from build123d import *

# Parameters (mm, degrees)
SKETCH_1_R          = 1.7
SKETCH_1_W          = 5
SKETCH_1_H          = 13
SKETCH_1_H_2        = 2
EXTRUDE_3_DEPTH     = 2.9
SKETCH_3_R          = 2.1
CUT_EXTRUDE_3_DEPTH = 2.9
SKETCH_4_W          = 20
SKETCH_4_H          = 40
SKETCH_4_R          = 2.1
EXTRUDE_4_DEPTH     = 2.9
SKETCH_5_W          = 70
SKETCH_5_H          = 40
SKETCH_5_W_2        = 69.6
SKETCH_5_H_2        = 39.6
CUT_EXTRUDE_4_DEPTH = 2.9


with BuildPart() as part:
    # 草图1 → 凸台-拉伸3 (new body)
    # profile 1 of 10: a face of its own
    with BuildSketch(Plane(origin=(0, 0, 0), x_dir=(1, 0, 0), z_dir=(0, 1, 0))):
        with BuildLine():
            Line((-40, 113), (-70, 113))
            Line((-70, 113), (-70, 108))
            Line((-70, 108), (-70, 92))
            Line((-70, 92), (-63.7, 92))
            ThreePointArc((-63.7, 92), (-62, 93.7), (-60.3, 92))
            ThreePointArc((-60.3, 92), (-60.797918472, 90.797918472), (-62, 90.3))
            Line((-62, 90.3), (-62, 87))
            Line((-62, 87), (-48, 87))
            Line((-48, 87), (-48, 90.3))
            ThreePointArc((-48, 90.3), (-49.202081528, 93.202081528), (-46.3, 92))
            Line((-46.3, 92), (-40, 92))
            Line((-40, 92), (-40, 113))
        make_face()
        with Locations(Location((-62, 108, 0), (0, 0, 270))):
            Circle(SKETCH_1_R, mode=Mode.SUBTRACT)
        with Locations(Location((-48, 108, 0), (0, 0, 270))):
            Circle(SKETCH_1_R, mode=Mode.SUBTRACT)
    # profile 2 of 10: a face of its own
    with BuildSketch(Plane(origin=(0, 0, 0), x_dir=(1, 0, 0), z_dir=(0, 1, 0))):
        with BuildLine():
            Line((-70, 92), (-70, 87))
            Line((-70, 87), (-62, 87))
            Line((-62, 87), (-62, 90.3))
            ThreePointArc((-62, 90.3), (-63.202081528, 90.797918472), (-63.7, 92))
            Line((-63.7, 92), (-70, 92))
        make_face()
    # profile 3 of 10: a face of its own
    with BuildSketch(Plane(origin=(0, 0, 0), x_dir=(1, 0, 0), z_dir=(0, 1, 0))):
        with BuildLine():
            Line((-48, 90.3), (-48, 87))
            Line((-48, 87), (-40, 87))
            Line((-40, 87), (-40, 92))
            Line((-40, 92), (-46.3, 92))
            ThreePointArc((-46.3, 92), (-46.797918472, 90.797918472), (-48, 90.3))
        make_face()
    # profile 4 of 10: a face of its own
    with BuildSketch(Plane(origin=(0, 0, 0), x_dir=(1, 0, 0), z_dir=(0, 1, 0))):
        Polygon((-70, 87), (-70, 80), (-20, 80), (-20, 85), (-25, 85), (-25, 87), (-40, 87), (-48, 87), (-62, 87), align=None)
    # profile 5 of 10: a face of its own
    with BuildSketch(Plane(origin=(0, 0, 0), x_dir=(1, 0, 0), z_dir=(0, 1, 0))):
        Polygon((-25, 113), (-40, 113), (-40, 92), (-40, 87), (-25, 87), (-25, 100), align=None)
    # profile 6 of 10: a face of its own
    with BuildSketch(Plane(origin=(0, 0, 0), x_dir=(1, 0, 0), z_dir=(0, 1, 0))):
        with Locations((-22.5, 93.5)):
            Rectangle(SKETCH_1_W, SKETCH_1_H)
    # profile 7 of 10: a face of its own
    with BuildSketch(Plane(origin=(0, 0, 0), x_dir=(1, 0, 0), z_dir=(0, 1, 0))):
        with Locations((-22.5, 106.5)):
            Rectangle(SKETCH_1_W, SKETCH_1_H)
    # profile 8 of 10: a face of its own
    with BuildSketch(Plane(origin=(0, 0, 0), x_dir=(1, 0, 0), z_dir=(0, 1, 0))):
        with Locations((-22.5, 86)):
            Rectangle(SKETCH_1_W, SKETCH_1_H_2)
    # profile 9 of 10: a face of its own
    with BuildSketch(Plane(origin=(0, 0, 0), x_dir=(1, 0, 0), z_dir=(0, 1, 0))):
        Polygon((-20, 120), (-70, 120), (-70, 113), (-40, 113), (-25, 113), (-25, 115), (-20, 115), align=None)
    # profile 10 of 10: a face of its own
    with BuildSketch(Plane(origin=(0, 0, 0), x_dir=(1, 0, 0), z_dir=(0, 1, 0))):
        with Locations((-22.5, 114)):
            Rectangle(SKETCH_1_W, SKETCH_1_H_2)
    extrude(amount=EXTRUDE_3_DEPTH)

    # 草图3 → 切除-拉伸3 (cut)
    with BuildSketch(Plane(origin=(0, 2.9, 0), x_dir=(1, 0, 0), z_dir=(0, 1, 0))):
        with Locations(Location((-25, 110, 0), (0, 0, 270))):
            Circle(SKETCH_3_R)
        with Locations(Location((-25, 90, 0), (0, 0, 270))):
            Circle(SKETCH_3_R)
        with Locations(Location((-35, 90, 0), (0, 0, 270))):
            Circle(SKETCH_3_R)
        with Locations(Location((-35, 110, 0), (0, 0, 270))):
            Circle(SKETCH_3_R)
    extrude(amount=-CUT_EXTRUDE_3_DEPTH, mode=Mode.SUBTRACT)

    # 草图4 → 凸台-拉伸4 (add)
    with BuildSketch(Plane(origin=(0, 2.9, 0), x_dir=(1, 0, 0), z_dir=(0, 1, 0))):
        with Locations((-10, 100)):
            Rectangle(SKETCH_4_W, SKETCH_4_H)
        with Locations(Location((-15, 110, 0), (0, 0, 270))):
            Circle(SKETCH_4_R, mode=Mode.SUBTRACT)
        with Locations(Location((-15, 90, 0), (0, 0, 270))):
            Circle(SKETCH_4_R, mode=Mode.SUBTRACT)
        with Locations(Location((-5, 110, 0), (0, 0, 270))):
            Circle(SKETCH_4_R, mode=Mode.SUBTRACT)
        with Locations(Location((-5, 90, 0), (0, 0, 270))):
            Circle(SKETCH_4_R, mode=Mode.SUBTRACT)
    extrude(amount=-EXTRUDE_4_DEPTH)

    # 草图5 → 切除-拉伸4 (cut)
    with BuildSketch(Plane(origin=(0, 2.9, 0), x_dir=(1, 0, 0), z_dir=(0, 1, 0))):
        with Locations((-35, 100)):
            Rectangle(SKETCH_5_W, SKETCH_5_H)
        with Locations((-35, 100)):
            Rectangle(SKETCH_5_W_2, SKETCH_5_H_2, mode=Mode.SUBTRACT)
    extrude(amount=-CUT_EXTRUDE_4_DEPTH, mode=Mode.SUBTRACT)


solid = part.part
CAD build for the part. Positions are in the model's coordinates, mm. Coordinates: 2 decimals unless noted, no trailing zeros. Order: outer loops, then holes, each group sorted by start corner. A loop starts at its lowest first (then second) coordinate and runs counter-clockwise, first axis right, second up.
Item 1: Two-plate mould, pull along X, no slides. Class faces 1 (the face through (-36.278, 1.47, -91.666)), 2 (the face through (-35, 2.9, -100)), 3 (the face through (-0.2, 1, -100)): +X half, -X half, draft (parallel to the pull), parting line (faces both ways), or undercut.
Check sheet entries:
face 1: undercut
face 2: draft
face 3: +X half
Item 2: Pin check, flat tip, straight feed: pin 1 Ø2.5 at (x, z) = (-5, -90) entering from -Y. Stop position of the tip, or through.
Check sheet entries:
pin 1: passes through
Item 3: Band-saw the part on A-A on z = -107. List the corners of the cut face in (x, y).
Check sheet entries:
outline: (-69.8, 0) - (-63.37, 0) - (-63.37, 2.9) - (-69.8, 2.9) - close; (-60.63, 0) - (-49.37, 0) - (-49.37, 2.9) - (-60.63, 2.9) - close; (-46.63, 0) - (-0.2, 0) - (-0.2, 2.9) - (-46.63, 2.9) - close
Item 4: Band-saw the part on C-C on y = 2.3. Give the number of separate pieces and of enclosed holes in the cut face, plus the area to 3 significant figures.
Check sheet entries:
separate pieces: 1
enclosed holes: 12
area: 2,610 mm2
Item 5: Band-saw the part on B-B on x = -35. List the corners of the cut face in (y, z).
Check sheet entries:
outline: (0, -119.8) - (2.9, -119.8) - (2.9, -112.1) - (0, -112.1) - close; (0, -107.9) - (2.9, -107.9) - (2.9, -92.1) - (0, -92.1) - close; (0, -87.9) - (2.9, -87.9) - (2.9, -80.2) - (0, -80.2) - close
Item 6: Drill centre lines: L1, parallel to X at y = 1, z = -90; L2, parallel to Z at x = -33.5, y = 0.5; L3, parallel to X at y = 2.6, z = -107. Where is each one in solid material? Low to high.
Check sheet entries:
L1: x = -69.8 to -37.1, -32.9 to -27.1, -22.9 to -17.1, -12.9 to -7.1, -2.9 to -0.2
L2: z = -119.8 to -111.47, -108.53 to -91.47, -88.53 to -80.2
L3: x = -69.8 to -63.37, -60.63 to -49.37, -46.63 to -0.2
